Study the drawing (mm; zero at the part's minimum x, y, z) and answer. A direction names the side the tool comes from. Give positions to 0.01 mm unless a question says otherwise; leave off trailing zeros. Order: outer loops, then holes, each group sorted by start corner. A loop starts at its lowest first (then second) coordinate and runs counter-clockwise, first axis right, second up. Notation, with made-up numbers: (66, 81.5) -> (111, 81.5) arc R26 ccw to (111, 95.5) -> close; hole circle Ø8 at (40.5, -38). An arc over 180 degrees is marked (long way). Answer as CSV lines item,"result". Start each with the question number.
1. A cutting plane is placed at D-D (z = 16). Give the vertices of the cut face in (x, y), then the cut area to 3 significant figures.
2. A cutting plane is placed at A-A (x = 39.9). Give the vertices of the cut face in (y, z).
3. For the marked faces 1 and 2, determine the directions among +Z, -Z, +X, -X, +Y, -Y from which every point of the face is accessible in a straight line to the end or side of a thin tool.
4. A cutting plane is placed at C-C (y = 8.5). Give the vertices of the cut face in (x, z).
5. For a pull along Z with two mould halves and no side action, classify the marked faces 3, 4, 5 and 6 as released by +Z, released by -Z, zero draft, split by the parting line, or undercut.
6. Flat-ended cylindrical pins translate along their axes: pin 1 (1 mm diameter, centred on x = 10.5, y = 16.5, fed in from +Z); pin 2 (25 mm diameter, centred on x = 16, z = 36, fed in from +Y). Find the tip coordinate at first contact, or state that the pin passes through.
7. A cutting plane is placed at B-B (y = 19.25). Give the vertices of the cut face in (x, z), then the cut area to 3 significant figures.
8. Find the intervals of material crossed by L1, parallel to X at y = 19, z = 65; L2, parallel to Z at x = 19.5, y = 4.5; L3, parallel to X at y = 32, z = 29, in increasing order.
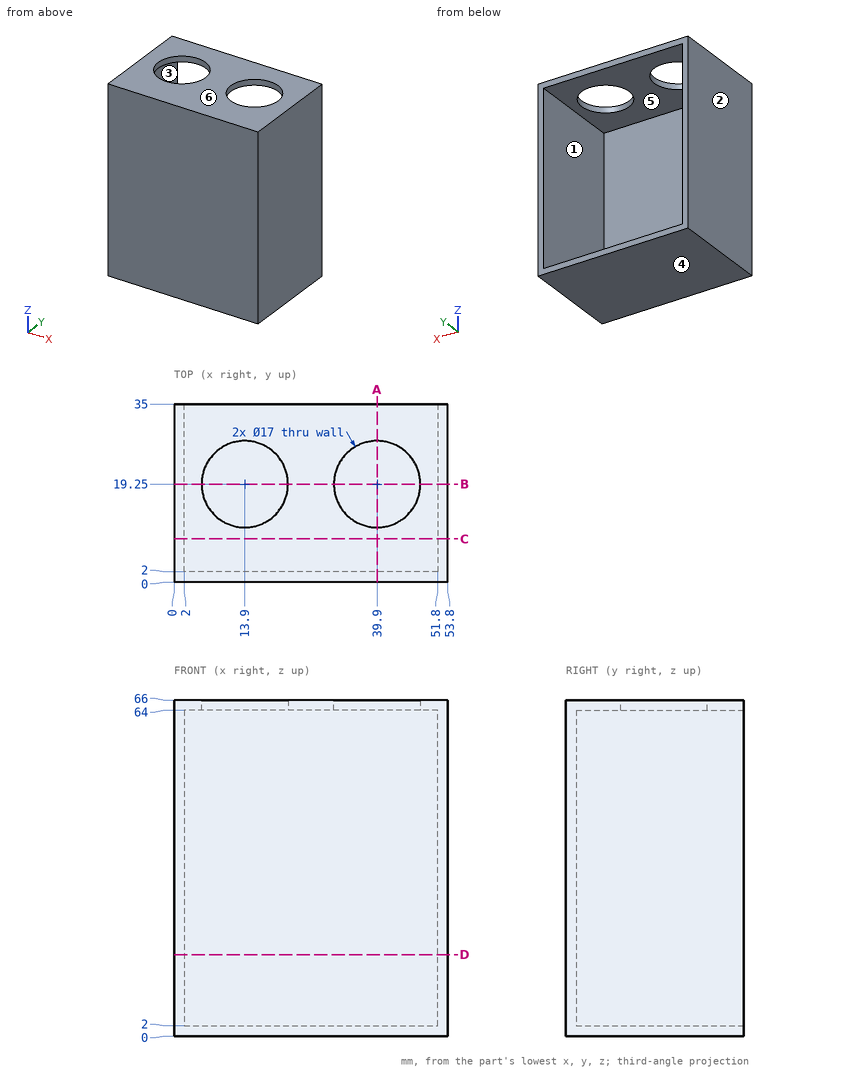
Answer sheet:
1,outline,"(0, 0) -> (53.8, 0) -> (53.8, 35) -> (51.8, 35) -> (51.8, 2) -> (2, 2) -> (2, 35) -> (0, 35) -> close"
1,area,"240 mm^2"
2,outline,"(0, 0) -> (35, 0) -> (35, 2) -> (2, 2) -> (2, 64) -> (10.75, 64) -> (10.75, 66) -> (0, 66) -> close; (27.75, 64) -> (35, 64) -> (35, 66) -> (27.75, 66) -> close"
3,face 1,"+Y"
3,face 2,"+Z, -Z, -X, +Y, -Y"
4,outline,"(0, 0) -> (53.8, 0) -> (53.8, 66) -> (0, 66) -> close; hole (2, 2) -> (51.8, 2) -> (51.8, 64) -> (2, 64) -> close"
5,face 3,"undercut"
5,face 4,"released by -Z"
5,face 5,"undercut"
5,face 6,"released by +Z"
6,pin 1,"stops at z = 2"
6,pin 2,"stops at y = 2"
7,outline,"(0, 0) -> (53.8, 0) -> (53.8, 66) -> (48.4, 66) -> (48.4, 64) -> (51.8, 64) -> (51.8, 2) -> (2, 2) -> (2, 64) -> (5.4, 64) -> (5.4, 66) -> (0, 66) -> close; (22.4, 64) -> (31.4, 64) -> (31.4, 66) -> (22.4, 66) -> close"
7,area,"395 mm^2"
8,L1,"x = 0 to 5.4, 22.4 to 31.4, 48.4 to 53.8"
8,L2,"z = 0 to 2, 64 to 66"
8,L3,"x = 0 to 2, 51.8 to 53.8"
